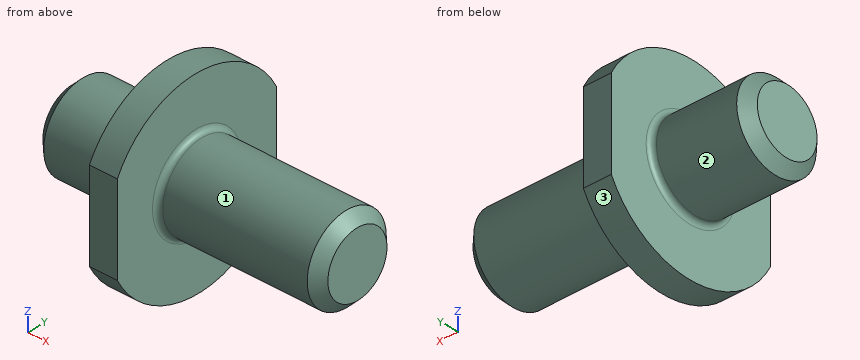
from build123d import *

# Parameters (mm, degrees)
CHAMFER1_SIZE           = 1
FILLET1_R               = 0.5
SKETCH2_OUTSIDE_W       = 27.366
SKETCH2_OUTSIDE_H       = 27.366
SKETCH2_OUTSIDE_W_2     = 26.756004186
SKETCH2_OUTSIDE_H_2     = 16
CUT_EXTRUDE1_DEPTH      = 18.61
CUT_EXTRUDE1_DEPTH_BACK = 10


with BuildPart() as part:
    # Sketch1 → Revolve1 (revolve)
    with BuildSketch(Plane.XY):
        Polygon((0, 4), (0, 9), (2.61, 9), (2.61, 3.96875), (17.61, 3.96875), (17.61, 0), (-9, 0), (-9, 4), align=None)
    revolve(axis=Axis((-38.174026976, 0, 0), (1, 0, 0)))

    # Chamfer1
    chamfer1_edges = [part.edges().sort_by_distance(p)[0] for p in [
        (17.61, -3.96875, 0),
        (-9, -4, 0),
    ]]
    chamfer(chamfer1_edges, length=CHAMFER1_SIZE)

    # Fillet1
    fillet1_edges = [part.edges().sort_by_distance(p)[0] for p in [
        (0, -4, 0),
        (2.61, -3.96875, 0),
    ]]
    fillet(fillet1_edges, radius=FILLET1_R)

    # Sketch2 outside → Cut-Extrude1 (cut, two sides)
    with BuildSketch(Plane(origin=(0, 0, 0), x_dir=(0, 0, -1), z_dir=(1, 0, 0))) as cut_extrude1_sk:
        Rectangle(SKETCH2_OUTSIDE_W, SKETCH2_OUTSIDE_H)
        Rectangle(SKETCH2_OUTSIDE_W_2, SKETCH2_OUTSIDE_H_2, mode=Mode.SUBTRACT)
    extrude(amount=CUT_EXTRUDE1_DEPTH, mode=Mode.SUBTRACT)
    extrude(cut_extrude1_sk.sketch, amount=-CUT_EXTRUDE1_DEPTH_BACK, mode=Mode.SUBTRACT)


solid = part.part
Geometry check sheet. Reference: the model listing, model coordinates, mm. Face numbers are marked on the shaded views. A direction names the side the tool comes from. Give positions to 0.01 mm unless a question says otherwise; leave off trailing zeros. Order: outer loops, then holes, each group sorted by start corner. A loop starts at its lowest first (then second) coordinate and runs counter-clockwise, first axis right, second up. Notation, with made-up numbers: M -29,76 L -9,76 A17 ccw -9,93 Z; hole C 73.5,73 d4. An arc over 180 degrees is marked long. Use a Markdown table: item, result.
Item 1: Section check D-D (x = -2.25). Record the cut outline in (y, z).
Answers follow:
| item | result |
|---|---|
| outline | C 0,0 d8 |
Item 2: Section check C-C (x = 11.5). Record the cut outline in (y, z), and give its area (3 significant figures).
Answers follow:
| item | result |
|---|---|
| outline | C 0,0 d7.94 |
| area | 49.5 mm2 |
Item 3: Depth check by flat-ended pin: P1, Ø1, axis at y = 4.5, z = -2, coming from the -X side; P2, Ø6, axis at x = -5.5, z = -1.5, coming from the +Y side; P3, Ø3, axis at y = 1.5, z = 5, coming from the +X side; P4, Ø6, axis at x = 0.5, z = -6, coming from the +Y side. Enter the tip coordinate at first touch or a pass-through.
Answers follow:
| item | result |
|---|---|
| P1 | stops at x = -0.01 |
| P2 | stops at y = 4 |
| P3 | stops at x = 16.86 |
| P4 | stops at y = 8 |
Item 4: Section check B-B (y = 0). Record the cut outline in (x, z).
Answers follow:
| item | result |
|---|---|
| outline | M -9,-3 L -8,-4 L -0.5,-4 A0.5 cw 0,-4.5 L 0,-9 L 2.61,-9 L 2.61,-4.47 A0.5 cw 3.11,-3.97 L 16.61,-3.97 L 17.61,-2.97 L 17.61,2.97 L 16.61,3.97 L 3.11,3.97 A0.5 cw 2.61,4.47 L 2.61,9 L 0,9 L 0,4.5 A0.5 cw -0.5,4 L -8,4 L -9,3 Z |
Item 5: Section check A-A (z = 0). Record the cut outline in (x, y), and give its area (3 significant figures).
Answers follow:
| item | result |
|---|---|
| outline | M -9,-3 L -8,-4 L -0.5,-4 A0.5 cw 0,-4.5 L 0,-8 L 2.61,-8 L 2.61,-4.47 A0.5 cw 3.11,-3.97 L 16.61,-3.97 L 17.61,-2.97 L 17.61,2.97 L 16.61,3.97 L 3.11,3.97 A0.5 cw 2.61,4.47 L 2.61,8 L 0,8 L 0,4.5 A0.5 cw -0.5,4 L -8,4 L -9,3 Z |
| area | 231 mm2 |
Item 6: Material ranges on line 1 along X through (y, z) = (-4.5, 2.25); line 2 along Y through (x, z) = (2, -4.5); line 3 along Z through (x, y) = (-3.75, 3), recorded low to high.
Answers follow:
| item | result |
|---|---|
| line 1 | x = 0 to 2.61 |
| line 2 | y = -7.79 to 7.79 |
| line 3 | z = -2.65 to 2.65 |
Item 7: Tool access check on the marked faces 1, 2 and 3. Record the directions out of +Z, -Z, +X, -X, +Y, -Y that give a thin tool (end or side, any length) a straight path to the whole face; none if there is none.
Answers follow:
| item | result |
|---|---|
| face 1 | +X |
| face 2 | -X |
| face 3 | -Z, +X, -X |
